from build123d import *

# Parameters (mm, degrees)
EXTRUDE_THIN1_DEPTH = 603.25
FILLET1_R           = 1.27


with BuildPart() as part:
    # Sketch1 → Extrude-Thin1 (new body)
    with BuildSketch(Plane.XY):
        with BuildLine():
            Line((0, 55.5625), (0, 60.325))
            Line((0, 60.325), (-17.4625, 60.325))
            ThreePointArc((-17.4625, 60.325), (-18.857403955, 56.957403955), (-22.225, 55.5625))
            Line((-22.225, 55.5625), (-22.225, 42.795329036))
            Line((-22.225, 42.795329036), (-19.05, 42.795329036))
            ThreePointArc((-19.05, 42.795329036), (-19.983849695, 35.617826147), (-16.845026643, 29.095831604))
            ThreePointArc((-16.845026643, 29.095831604), (-11.927389151, 19.928241149), (-11.90625, 9.525))
            Line((-11.90625, 9.525), (-7.9375, 9.525))
            Line((-7.9375, 9.525), (-7.9375, 0))
            Line((-7.9375, 0), (0, 0))
            Line((0, 0), (0, 4.7625))
            Line((0, 4.7625), (-1.27, 4.7625))
            Line((-1.27, 4.7625), (-1.27, 1.27))
            Line((-1.27, 1.27), (-6.6675, 1.27))
            Line((-6.6675, 1.27), (-6.6675, 10.795))
            Line((-6.6675, 10.795), (-10.341607608, 10.795))
            ThreePointArc((-10.341607608, 10.795), (-10.90685332, 21.016186768), (-15.905046277, 29.949843847))
            ThreePointArc((-15.905046277, 29.949843847), (-18.847187578, 36.835889429), (-16.895515947, 44.065329036))
            Line((-16.895515947, 44.065329036), (-20.955, 44.065329036))
            Line((-20.955, 44.065329036), (-20.955, 54.42769924))
            ThreePointArc((-20.955, 54.42769924), (-17.959378342, 56.059378342), (-16.32769924, 59.055))
            Line((-16.32769924, 59.055), (-1.27, 59.055))
            Line((-1.27, 59.055), (-1.27, 55.5625))
            Line((-1.27, 55.5625), (0, 55.5625))
        make_face()
    extrude(amount=-EXTRUDE_THIN1_DEPTH)

    # Fillet1
    fillet1_edges = [part.edges().sort_by_distance(p)[0] for p in [
        (0, 0, -301.625),
        (-7.9375, 0, -301.625),
        (-11.90625, 9.525, -301.625),
        (-22.225, 42.795329036, -301.625),
        (-22.225, 55.5625, -301.625),
        (-17.4625, 60.325, -301.625),
        (0, 60.325, -301.625),
        (-16.895515947, 44.065329036, -301.625),
        (-6.6675, 10.795, -301.625),
    ]]
    fillet(fillet1_edges, radius=FILLET1_R)


solid = part.part
CAD build for the part. Positions are in the model's coordinates, mm. A direction names the side the tool comes from. Round coordinates to 2 decimals unless told otherwise and drop trailing zeros. Order: outer loops, then holes, each group sorted by start corner. A loop starts at its lowest first (then second) coordinate and runs counter-clockwise, first axis right, second up. Notation, with made-up numbers: (-30.75, 32.5) -> (16.25, 32.5) arc R21 cw to (16.25, 67.5) -> close; hole circle Ø11 at (49.25, -22). An arc over 180 degrees is marked (long way). Write item = value, one per line. Start each with the question number.
(1) Cut at B-B, the plane y = 37. List the corners of the cut face in (x, z).
(2) Probe line 1 (Y direction, x = -5, z = -52.5) (3 decimals); line 2 (X direction, y = 4.5, z = -339); line 3 (Y direction, x = -8.75, z = -138) (3 decimals). List the from-to ranges inside material, lowest first. Write a range as [from, to].
(3) Pull direction Y, two halves, no side cores. Call faces 4 (the flat face through (-9, 60.325, -297)), 5 (the flat face through (-22.225, 49, -297)), 6 (the cylindrical face through (-12.165, 20.793, -297.402)): released by +Y, released by -Y, zero draft, split by the parting line, or undercut.
(4) Pin check, flat tips, straight feed: P1, Ø1, axis at x = -0.5, z = -384, coming from the +Y side; P2, Ø2.5, axis at y = 4, z = -346, coming from the -X side; P3, Ø0.6, axis at x = -20, z = -288, coming from the +Y side; P4, Ø0.6, axis at x = -1, z = -248.5, coming from the -Y side. Stop position of each tip, or through.
(5) Which spindle directions (+Z, -Z, +X, -X, +Y, -Y) get a long thin tool onto all of the face, cutting with end or side? Do faces 1 (the flat face through (-20.955, 49, -297)), 2 (the flat face through (-17, 30, -603.25)), 3 (the flat face through (-9, 59.055, -297)). Say none if no direction does.
Model answer:
q1.outline = (-20.13, -603.25) -> (-18.86, -603.25) -> (-18.86, 0) -> (-20.13, 0) -> close
q2.line_1 = [0, 1.27], [59.055, 60.325]
q2.line_2 = [-7.94, -6.67], [-1.27, 0]
q2.line_3 = [9.525, 10.795], [59.055, 60.325]
q3.face_4 = released by +Y
q3.face_5 = zero draft
q3.face_6 = undercut
q4.P1 = 60.3
q4.P2 = -7.94
q4.P3 = 56.29
q4.P4 = 0
q5.face_1 = +Z, -Z, +X
q5.face_2 = -Z, +X, -X, +Y, -Y
q5.face_3 = +Z, -Z
